Check sheet for the modelled part. Datum: model origin and axes. Units: mm. Face numbers are marked on the shaded views. A direction names the side the tool comes from. Coordinates: 2 decimals unless noted, no trailing zeros. Loops run counter-clockwise (first coordinate to the right, second up) from the corner with the lowest first, then second, coordinate; pieces in that order, holes last. Notation, with made-up numbers: (31.5, 8) - (78.5, 8) arc R15 ccw to (78.5, 15) - close; hole circle Ø4 at (-10.5, 35). An arc over 180 degrees is marked (long way). Write each question's results on one line, items separated by ' | '. Start each with the question number.
1. Cross-section at D-D (y = 3.75). Record the cut outline in (x, z), and give its area (3 significant figures).
2. Cross-section at B-B (x = -1). Record the cut outline in (y, z), and give its area (3 significant figures).
3. Cross-section at C-C (z = 9.5). Record the cut outline in (x, y), and give its area (3 significant figures).
4. Cross-section at A-A (y = 0). Record the cut outline in (x, z).
5. Tool access check on the marked faces 4 and 5. Record the directions out of +Z, -Z, +X, -X, +Y, -Y that give a thin tool (end or side, any length) a straight path to the whole face; none if there is none.
6. Gauge pin test, flat ends, axial feed: P1, Ø10, axis at x = -5.5, z = 6, coming from the -Y side; P2, Ø1.5, axis at y = 6.5, z = 7, coming from the +X side; P3, Ø6, axis at x = 7.5, y = 7.5, coming from the -Z side. Record the tip position at first contact, or that the pin passes through.
7. Thickness scan on line 1 (Y direction, x = 0, z = 3.5); line 2 (Y direction, x = -2.25, z = -3.5); line 3 (X direction, y = -2.5, z = 6.5). Record the ranges inside material, lowest first. Write a range as [from, to].
8. Draft check along X on the marked faces 1, 2 and 3. Enter one of: released by +X, released by -X, zero draft, split by the parting line, or undercut.
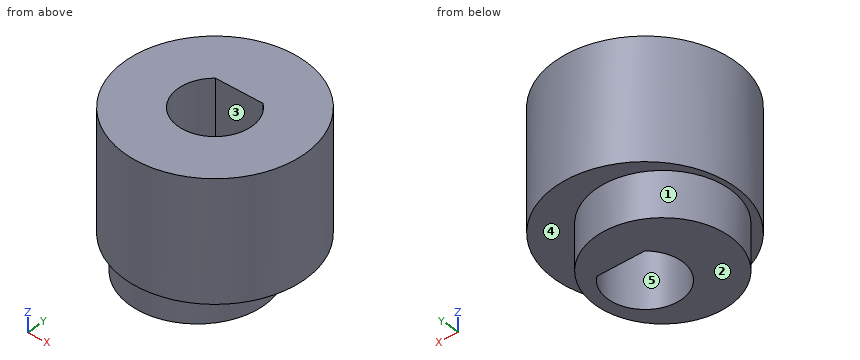
Autodesk Inventor part; units mm, degrees
ref_plane "YZ Plane" through (0, 0, 0) normal (1, 0, 0) x (0, 1, 0)
ref_plane "XZ Plane" through (0, 0, 0) normal (0, 1, 0) x (-1, 0, 0)
ref_plane "XY Plane" through (0, 0, 0) normal (0, 0, 1) x (1, 0, 0)
sketch "스케치1" plane through (0, 0, 0) normal (0, 0, 1) x (1, 0, 0)
  circle A0 centre (0, 0) radius 10
  circle A1 centre (0, 0) radius 4
  dimension "d0" = 20
  dimension "d1" = 8
extrude "돌출1" add sketch "스케치1" along normal blind 13.3
sketch "스케치2" plane through (0, 0, 0) normal (0, 0, -1) x (-1, 0, 0)
  line L0 (-2.6458, 3) -> (2.6458, 3)
  circle A0 centre (0, 0) radius 4
  dimension "d4" = 3
extrude "돌출2" add sketch "스케치2" against normal up to surface (13.3 mm away) contours A0 L0 picked at (-0.6179, 3.1815)
sketch "스케치3" plane through (0, 0, 0) normal (0, 0, -1) x (-1, 0, 0)
  circle A0 centre (2, 0) radius 7.45
  line L0 (0, 0) -> (2, 0)
  arc A1 (-2.6458, 3) -> (2.6458, 3) centre (0, 0) ccw
  line L1 (-2.6458, 3) -> (2.6458, 3)
  dimension "d7" = 14.9
  dimension "d8" = 2
extrude "돌출3" add sketch "스케치3" along normal blind 5
sketch "스케치4" plane through (-2, 0, -5) normal (0, 0, -1) x (-1, 0, 0)
  arc A0 (-4.6458, 3) -> (0.6458, 3) centre (-2, 0) ccw
  line L0 (-4.6458, 3) -> (0.6458, 3)
  arc A1 (-4.6833, 3.1) -> (0.6833, 3.1) centre (-2, 0) ccw
  line L1 (-4.6833, 3.1) -> (0.6833, 3.1)
  dimension "d11" = 0.1
extrude "돌출4" cut sketch "스케치4" against normal up to surface (18.3 mm away) contours L0 A0 | L1 A1
properties part number "감속기어1 - 축"
Established:
1) outline: (-9.27, 0) - (-8.44, 0) - (-8.44, -5) - (4.44, -5) - (4.44, 0) - (9.27, 0) - (9.27, 13.3) - (-9.27, 13.3) - close | area: 311 mm^2
2) outline: (-9.95, 0) - (-7.38, 0) - (-7.38, -5) - (-3.98, -5) - (-3.98, 13.3) - (-9.95, 13.3) - close; (3.1, -5) - (7.38, -5) - (7.38, 0) - (9.95, 0) - (9.95, 13.3) - (3.1, 13.3) - close | area: 209 mm^2
3) outline: circle Ø20 at (0, 0); hole (-2.68, 3.1) arc R4.1 ccw (long way) to (2.68, 3.1) - close | area: 265 mm^2
4) outline: (-10, 0) - (-9.45, 0) - (-9.45, -5) - (-4.1, -5) - (-4.1, 13.3) - (-10, 13.3) - close; (4.1, -5) - (5.45, -5) - (5.45, 0) - (10, 0) - (10, 13.3) - (4.1, 13.3) - close
5) face 4: -Z | face 5: +Z, -Z
6) P1: y = -9.99 | P2: x = 8.18 | P3: z = 0
7) line 1: [-10, -4.1], [3.1, 10] | line 2: [-7.45, -3.43], [3.1, 7.45] | line 3: [-9.68, -3.25], [3.25, 9.68]
8) face 1: split by the parting line | face 2: zero draft | face 3: undercut
